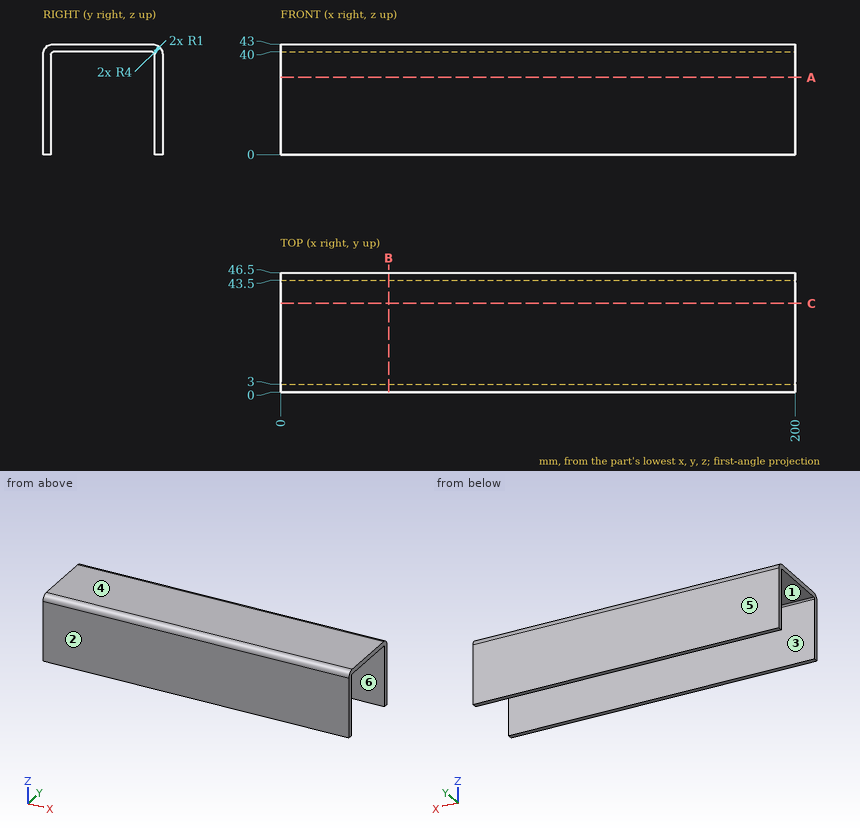
Design review of the part shown in the three views and the two pictorial views. Dimensions are in mm from the part's minimum x, y and z. A direction names the side the tool comes from. Give positions to 0.01 mm unless a question says otherwise; leave off trailing zeros. Order: outer loops, then holes, each group sorted by start corner. A loop starts at its lowest first (then second) coordinate and runs counter-clockwise, first axis right, second up. Notation, with made-up numbers: M 13,66 L 61,66 A24 cw 61,76 Z; hole C -12.5,40.5 d9. An arc over 180 degrees is marked long. Answer in a Markdown table with one row per item. Add a question column.
(1) For pin 1 (12 mm diameter, centred on x = 179, z = 26, fed in from -Y); pin 2 (6 mm diameter, centred on x = 95.5, y = 13.5, fed in from -Z), all flat-tipped, find the tip position at first contact; note any pin that passes through.
(2) Consider section A-A on z = 30. State the section outline as (x, y) points, and give its area (3 significant figures).
(3) For the marked faces 1 and 2, list the 3-axis set-ups (+Z, -Z, +X, -X, +Y, -Y) from which the entire face can be reached by the end or side of a thin tool; tool diameter is ignored.
(4) Consider section C-C on y = 34.5. State the section outline as (x, z) points, and give its area (3 significant figures).
(5) Mouldability with a two-part tool opening along Y and no side actions: class the marked faces 3, 4, 5 and 6 as +Y half, -Y half, draft (parallel to the pull), parting line (faces both ways), or undercut.
(6) Wall thickness on probe 1 along Y at (x, z) = (177, 20.5); probe 2 along Z at (x, y) = (68, 29.5); probe 3 along Y at (x, z) = (148.5, 39.5): over which ranges is each line inside the solid? List them lowest first. Write a range as [from, to].
(7) Consider section B-B on x = 42. State the section outline as (y, z) points.
Evaluation:
| question | item | result |
|---|---|---|
| 1 | pin 1 | stops at y = 0 |
| 1 | pin 2 | stops at z = 40 |
| 2 | outline | M 0,0 L 200,0 L 200,3 L 0,3 Z; M 0,43.5 L 200,43.5 L 200,46.5 L 0,46.5 Z |
| 2 | area | 1,200 mm^2 |
| 3 | face 1 | -Z, +X, -X |
| 3 | face 2 | +Z, -Z, +X, -X, -Y |
| 4 | outline | M 0,40 L 200,40 L 200,43 L 0,43 Z |
| 4 | area | 600 mm^2 |
| 5 | face 3 | undercut |
| 5 | face 4 | draft |
| 5 | face 5 | +Y half |
| 5 | face 6 | undercut |
| 6 | probe 1 | y = [0, 3], [43.5, 46.5] |
| 6 | probe 2 | z = [40, 43] |
| 6 | probe 3 | y = [0.03, 3.13], [43.37, 46.47] |
| 7 | outline | M 0,0 L 3,0 L 3,39 A1 cw 4,40 L 42.5,40 A1 cw 43.5,39 L 43.5,0 L 46.5,0 L 46.5,39 A4 ccw 42.5,43 L 4,43 A4 ccw 0,39 Z |
